Answer from the drawing. Dimensions are ordinates in mm from the lowest x, y and z of the part. Give positions to 0.01 mm unless a question says otherwise; leave off trailing zeros. Order: outer loops, then holes, each group sorted by start corner. A loop starts at its lowest first (then second) coordinate and runs counter-clockwise, first axis right, second up.
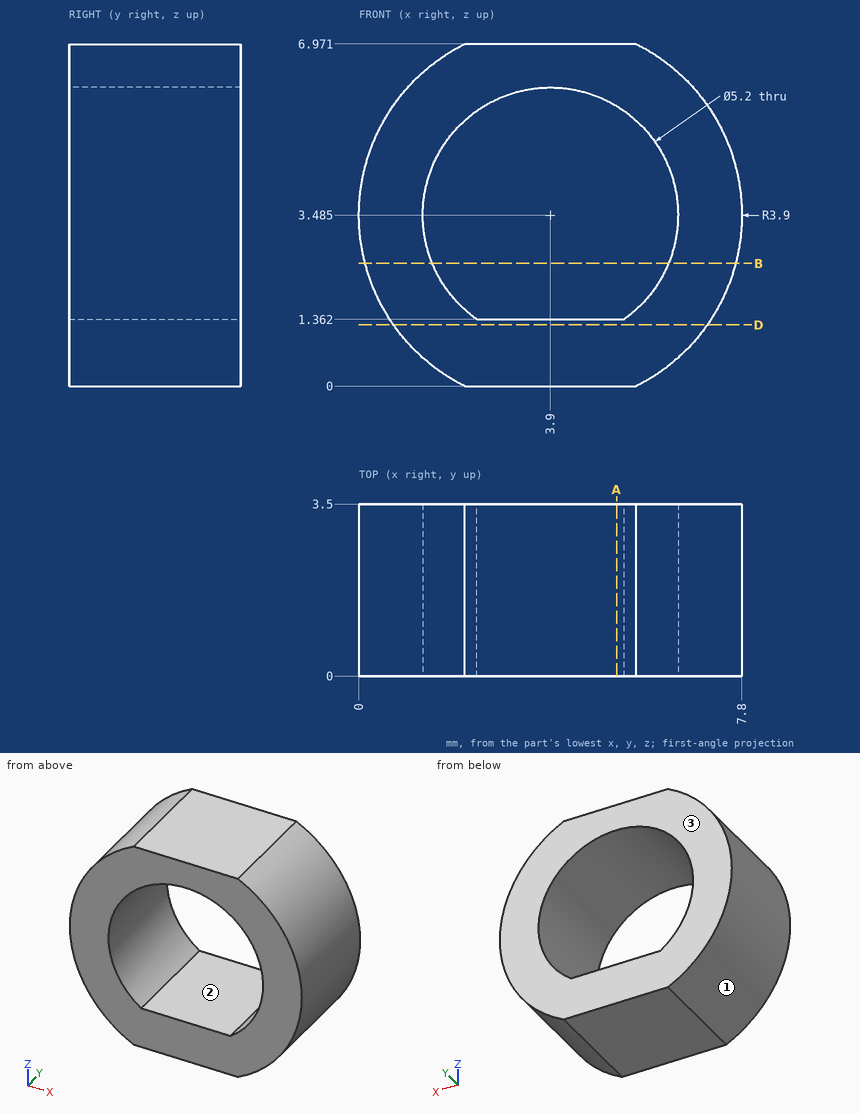
1) The part is cut by section D-D on z = 1.25. Determine the outline of the cut face in (x, y) (1 decimal).
Final values:
outline: (0.7, 0) - (7.1, 0) - (7.1, 3.5) - (0.7, 3.5) - close
2) Given pin 1 (1 mm diameter, centred on y = 2, z = 1, fed in from -X); pin 2 (1.5 mm diameter, centred on x = 4, y = 1, fed in from -Z), each flat-ended and moving along its own axis, determine where each tip first touches the part or whether it passes through.
Final values:
pin 1: stops at x = 0.54
pin 2: stops at z = 0
3) The part is cut by section B-B on z = 2.5. Determine the outline of the cut face in (x, y).
Final values:
outline: (0.13, 0) - (1.49, 0) - (1.49, 3.5) - (0.13, 3.5) - close; (6.31, 0) - (7.67, 0) - (7.67, 3.5) - (6.31, 3.5) - close
4) The part is cut by section A-A on x = 5.25. Determine the outline of the cut face in (y, z).
Final values:
outline: (0, 0) - (3.5, 0) - (3.5, 1.36) - (0, 1.36) - close; (0, 5.71) - (3.5, 5.71) - (3.5, 6.97) - (0, 6.97) - close
5) For a pull along Z with two mould halves and no side action, classify the marked faces 1, 2 and 3 as released by +Z, released by -Z, zero draft, split by the parting line, or undercut.
Final values:
face 1: split by the parting line
face 2: undercut
face 3: zero draft
6) Consider L1, parallel to X at y = 2.1, z = 1.5 (1 decimal); L2, parallel to X at y = 2.75, z = 5.25; L3, parallel to Z at x = 2.75, y = 0.6. Determine where each line is inside the solid, lowest interval first.
Final values:
L1: x = 0.5 to 2.2, 5.6 to 7.3
L2: x = 0.42 to 1.99, 5.81 to 7.38
L3: z = 0 to 1.36, 5.82 to 6.97
